Input: part model. Units: mm. Frame: model coordinates. A direction names the side the tool comes from. Give positions to 0.01 mm unless a question says otherwise; leave off trailing zeros. Write each loop counter-clockwise with the first axis right and the second up, starting at its lowest first coordinate (ties: lowest second). Pieces come first, ordered by that corner, then holes. Notation, with made-up numbers: (74.25, -39) -> (97.25, -39) arc R6 ccw to (97.25, -35) -> close; hole circle Ø10 at (89, 22). An arc over 180 degrees is marked (long way). Return JSON: item names as keys, results as strings. Group by question number.
Item 1: Pin query (flat end, axial travel): P1, Ø0.8, axis at x = 26.5, z = 33.5, coming from the +Y side; P2, Ø1.5, axis at x = 26.5, y = -25.5, coming from the -Z side; P3, Ø14.5, axis at y = -18.5, z = 16.5, coming from the -X side. Return the tip coordinate at first contact, or that it passes through.
Item 2: Section D-D, the plane x = 28. Return loops of the section in (y, z), then the cut area to 3 significant figures.
Item 3: Set-up query: faces 1 (the face through (34.95, -20, 19)), 2 (the face through (26, -5, 19)), 3 (the face through (21, -2, 33)). Return all of +Z, -Z, +X, -X, +Y, -Y with unobstructed straight access to the full face (end or side cutting, diameter ignored); none if empty.
Item 4: Section A-A, the plane y = -8.5. Return loops of the section in (x, z) (3 decimals), then the cut area to 3 significant figures.
Item 5: Mould query, pull axis Y, two halves, no side actions, for faces 4 (the face through (5.79, -6.89, 1.52)), 5 (the face through (25.6, -5, 33.5)), 6 (the face through (19, -35, 20)). Classes: released by +Y, released by -Y, zero draft, split by the parting line, or undercut.
Item 6: Section B-B, the plane x = 6. Return loops of the section in (y, z) (3 decimals), then the cut area to 3 significant figures.
Item 7: Line query: line 1 (Z direction, x = 28.5, y = -13.5); line 2 (Y direction, x = 36, z = 2) (3 decimals); line 3 (X direction, y = -12.5, z = 20.5). Output: solid intervals per line, ascending. Write a range as [from, to].
Item 8: Section C-C, the plane y = -23.5. Return loops of the section in (x, z), then the cut area to 3 significant figures.
from build123d import *

# Parameters (mm, degrees)
ESQUISSE1_W             = 42
ESQUISSE1_H             = 17
BOSS_EXTRU_1_DEPTH      = 3
ESQUISSE2_R             = 1.625
ENL_V_MAT_EXTRU_1_DEPTH = 4
ESQUISSE3_W             = 42
ESQUISSE3_H             = 5
BOSS_EXTRU_2_DEPTH      = 30
ESQUISSE4_W             = 18.4
ESQUISSE4_H             = 29.2
ESQUISSE4_W_2           = 12.4
ESQUISSE4_H_2           = 23.2
BOSS_EXTRU_3_DEPTH      = 30


with BuildPart() as part:
    # Esquisse1 → Boss.-Extru.1 (new body)
    with BuildSketch(Plane.XY):
        with Locations((21, -8.5)):
            Rectangle(ESQUISSE1_W, ESQUISSE1_H)
    extrude(amount=BOSS_EXTRU_1_DEPTH)

    # Esquisse2 → Enlèv. mat.-Extru.1 (cut, through all)
    with BuildSketch(Plane.XY.offset(3)):
        with Locations((6, -8.5)):
            Circle(ESQUISSE2_R)
        with Locations((36, -8.5)):
            Circle(ESQUISSE2_R)
    extrude(amount=-ENL_V_MAT_EXTRU_1_DEPTH, mode=Mode.SUBTRACT)

    # Esquisse3 → Boss.-Extru.2 (add)
    with BuildSketch(Plane.XY.offset(3)):
        with Locations((21, -2.5)):
            Rectangle(ESQUISSE3_W, ESQUISSE3_H)
    extrude(amount=BOSS_EXTRU_2_DEPTH)

    # Esquisse4 → Boss.-Extru.3 (add)
    with BuildSketch(Plane.XZ.offset(5)):
        with Locations((25.749828538, 19.382668745)):
            Rectangle(ESQUISSE4_W, ESQUISSE4_H)
        with Locations((25.749828538, 19.382668745)):
            Rectangle(ESQUISSE4_W_2, ESQUISSE4_H_2, mode=Mode.SUBTRACT)
    extrude(amount=BOSS_EXTRU_3_DEPTH)


solid = part.part
Answer below:
{
 "1": {"P1": "stops at y = -5", "P2": "stops at z = 4.78", "P3": "stops at x = 16.55"},
 "2": {"outline": "(-35, 4.78) -> (-5, 4.78) -> (-5, 3) -> (-17, 3) -> (-17, 0) -> (0, 0) -> (0, 33) -> (-5, 33) -> (-5, 33.98) -> (-35, 33.98) -> (-35, 30.98) -> (-5, 30.98) -> (-5, 7.78) -> (-35, 7.78) -> close", "area": "381 mm2"},
 "3": {"face 1": "+Z, +X, -Y", "face 2": "-Y", "face 3": "+Z, +X, -X, +Y"},
 "4": {"outline": "(0, 0) -> (4.375, 0) -> (4.375, 3) -> (0, 3) -> close; (7.625, 0) -> (34.375, 0) -> (34.375, 3) -> (7.625, 3) -> close; (16.55, 4.783) -> (34.95, 4.783) -> (34.95, 33.983) -> (16.55, 33.983) -> close; (37.625, 0) -> (42, 0) -> (42, 3) -> (37.625, 3) -> close; hole (19.55, 7.783) -> (31.95, 7.783) -> (31.95, 30.983) -> (19.55, 30.983) -> close", "area": "356 mm2"},
 "5": {"face 4": "undercut", "face 5": "released by +Y", "face 6": "released by -Y"},
 "6": {"outline": "(-17, 0) -> (-10.125, 0) -> (-10.125, 3) -> (-17, 3) -> close; (-6.875, 0) -> (0, 0) -> (0, 33) -> (-5, 33) -> (-5, 3) -> (-6.875, 3) -> close", "area": "191 mm2"},
 "7": {"line 1": "z = [0, 3], [4.78, 7.78], [30.98, 33.98]", "line 2": "y = [-17, -10.125], [-6.875, 0]", "line 3": "x = [16.55, 19.55], [31.95, 34.95]"},
 "8": {"outline": "(16.55, 4.78) -> (34.95, 4.78) -> (34.95, 33.98) -> (16.55, 33.98) -> close; hole (19.55, 7.78) -> (31.95, 7.78) -> (31.95, 30.98) -> (19.55, 30.98) -> close", "area": "250 mm2"}
}
